Input: part model. Units: mm. Frame: model coordinates. A direction names the side the tool comes from. Coordinates: 2 decimals unless noted, no trailing zeros. Loops run counter-clockwise (first coordinate to the right, second up) from the corner with the lowest first, then second, coordinate; pieces in that order, holes last.
(1) Contact query for flat-ended pins moving along their axis: P1, Ø2, axis at x = 15, z = 1, coming from the +Y side; P2, Ø1.5, axis at x = 11, z = 0.5, coming from the -Y side; P3, Ø1.5, axis at x = -8, z = 1, coming from the +Y side. Output: stop coordinate, or through.
(2) Line query: L1, parallel to X at y = 403, z = 0; L2, parallel to Y at x = 0, z = 3.5; L3, parallel to X at y = 617.5, z = -0.25. Output: solid intervals per line, ascending.
(3) Section B-B, the plane y = 189.5. Return loops of the section in (x, z).
(4) Set-up query: faces 1 (the face through (-0.42, 920.96, 0.05)), 2 (the face through (20, 453, -3.899)). Return all of +Z, -Z, +X, -X, +Y, -Y with unobstructed straight access to the full face (end or side cutting, diameter ignored); none if empty.
(5) Section A-A, the plane x = 0. Return loops of the section in (y, z).
(6) Mould query, pull axis X, two halves, no side actions, for faces 3 (the face through (20, 453, 3.899)), 4 (the face through (0.42, -19.26, 0.05)), 5 (the face through (-0.553, -25.153, 0.055)). Classes: released by +X, released by -X, zero draft, split by the parting line, or undercut.
```python
from build123d import *

# Parameters (mm, degrees)
BOSS_EXTRUDE1_DEPTH = 3.8989


with BuildPart() as part:
    # Sketch1 → Boss-Extrude1 (new body, symmetric)
    with BuildSketch(Plane.XY):
        with BuildLine():
            Line((-25.1587, 901.7), (-25.1587, 647.7))
            Line((-25.1587, 647.7), (-19.2659, 647.7))
            Line((-19.2659, 647.7), (-19.2659, 901.7))
            ThreePointArc((-19.2659, 901.7), (0, 920.9659), (19.2659, 901.7))
            Line((19.2659, 901.7), (19.2659, 0))
            ThreePointArc((19.2659, 0), (0, -19.2659), (-19.2659, 0))
            Line((-19.2659, 0), (-19.2659, 600.075))
            Line((-19.2659, 600.075), (-25.1587, 600.075))
            Line((-25.1587, 600.075), (-25.1587, 0))
            ThreePointArc((-25.1587, 0), (0, -25.1587), (25.1587, 0))
            Line((25.1587, 0), (25.1587, 901.7))
            ThreePointArc((25.1587, 901.7), (0, 926.8587), (-25.1587, 901.7))
        make_face()
    extrude(amount=BOSS_EXTRUDE1_DEPTH, both=True)


solid = part.part
```
Report:
1. P1: stops at y = 922.6
1. P2: stops at y = -22.98
1. P3: stops at y = 925.79
2. L1: x = -25.16 to -19.27, 19.27 to 25.16
2. L2: y = -25.16 to -19.27, 920.97 to 926.86
2. L3: x = 19.27 to 25.16
3. outline: (-25.16, -3.9) - (-19.27, -3.9) - (-19.27, 3.9) - (-25.16, 3.9) - close; (19.27, -3.9) - (25.16, -3.9) - (25.16, 3.9) - (19.27, 3.9) - close
4. face 1: +Z, -Z
4. face 2: -Z, +X, -X, +Y, -Y
5. outline: (-25.16, -3.9) - (-19.27, -3.9) - (-19.27, 3.9) - (-25.16, 3.9) - close; (920.97, -3.9) - (926.86, -3.9) - (926.86, 3.9) - (920.97, 3.9) - close
6. face 3: zero draft
6. face 4: undercut
6. face 5: split by the parting line
